Here's how the part is built. I have some questions about the finished solid (model axes, mm). A direction names the side the tool comes from. Round coordinates to 2 decimals unless told otherwise and drop trailing zeros. Order: outer loops, then holes, each group sorted by start corner. A loop starts at its lowest first (then second) coordinate and runs counter-clockwise, first axis right, second up. Notation, with made-up numbers: (61, -7.5) -> (95, -7.5) arc R30 ccw to (95, 14.5) -> close; hole circle Ø11 at (84.25, -24.75). An arc over 180 degrees is marked (long way). Answer in a Markdown table with one row per item.
```python
from build123d import *

# Parameters (mm, degrees)
F0_W     = 101.1391505599
F0_H     = 70.6634148955
F1_DEPTH = 6.35
F2_W     = 3.4494325519
F2_H     = 70.6634148955
F3_DEPTH = 59.06905
F3_TAPER = 1


with BuildPart() as f1:
    # F0 (on Front) → F1 (new body)
    with BuildSketch(Plane.XZ):
        Rectangle(F0_W, F0_H)
    extrude(amount=F1_DEPTH)

    # F2 (on face) → F3 (join)
    with BuildSketch(Plane.XZ.offset(6.35)):
        with Locations((-48.844859004, 0)):
            Rectangle(F2_W, F2_H)
    extrude(amount=F3_DEPTH, taper=F3_TAPER)


solid = f1.part
```
1. For pin 1 Ø8 at (y, z) = (-14.5, -27.5) entering from -X; pin 2 Ø1 at (y, z) = (-45, -27.5) entering from +X; pin 3 Ø5 at (y, z) = (-58.5, -23.5) entering from +X, each with a flat end and sliding along its axis, tell me the tip position at first contact or that it passes through.
Numbers:
| item | result |
|---|---|
| pin 1 | stops at x = -50.5 |
| pin 2 | stops at x = -47.79 |
| pin 3 | stops at x = -47.99 |
2. Suppose I cut it at A-A on x = 40.5. Write out the boundary of the cut face in (y, z), then the cut area to 3 significant figures.
Numbers:
| item | result |
|---|---|
| outline | (-6.35, -35.33) -> (0, -35.33) -> (0, 35.33) -> (-6.35, 35.33) -> close |
| area | 449 mm2 |
3. Please list where these lines run through material, in increasing order: line 1 along Y through (x, z) = (-42.5, -12.5); line 2 along X through (y, z) = (-26, -12); line 3 along X through (y, z) = (-45, 30).
Numbers:
| item | result |
|---|---|
| line 1 | y = -6.35 to 0 |
| line 2 | x = -50.23 to -47.46 |
| line 3 | x = -49.89 to -47.79 |
4. For faces 1 (the face through (-1, -3, -35.332)), 2 (the face through (1, -6.35, 0)), which set-ups out of +Z, -Z, +X, -X, +Y, -Y let a thin tool reach every point of the face, with its end or its side?
Numbers:
| item | result |
|---|---|
| face 1 | -Z, +X, -X, +Y, -Y |
| face 2 | +Z, -Z, +X, -Y |
